Source: CAD feature listing. Evaluate the final solid. Frame: model axes, mm. Face numbers are marked on the shaded views. A direction names the side the tool comes from. Give positions to 0.01 mm unless a question says otherwise; leave off trailing zeros. Order: outer loops, then holes, each group sorted by start corner. A loop starts at its lowest first (then second) coordinate and runs counter-clockwise, first axis right, second up. Notation, with made-up numbers: M 78.5,-13.5 L 94.5,-13.5 A37 cw 94.5,24.5 Z; hole C 49,0 d8. An arc over 180 degrees is marked long. Answer as a JSON object with one key per item and string values. Group by question number.
1. Pin query (flat end, axial travel): P1, Ø2, axis at x = -6.5, y = 9.5, coming from the +Z side; P2, Ø4, axis at y = 6, z = 14, coming from the +X side; P3, Ø1, axis at x = -8, z = 10.5, coming from the +Y side. Return the tip coordinate at first contact, or that it passes through.
2. Set-up query: the marked faces 4 and 5. Return all of +Z, -Z, +X, -X, +Y, -Y with unobstructed straight access to the full face (end or side cutting, diameter ignored); none if empty.
3. Section query D-D (x = -18). Output: boundary loops of the cut face in (y, z).
4. Section query A-A (y = 0). Output: boundary loops of the cut face in (x, z), plus the area to 4 significant figures.
5. Material intervals for L1, parallel to Y at x = 0, z = 5.5; L2, parallel to Z at x = 0, y = -5; L3, parallel to Z at x = -7.5, y = -7, sorted ascending. Write a range as [from, to].
6. Section query C-C (z = 16.75). Output: boundary loops of the cut face in (x, y), plus the area to 3 significant figures.
7. Pull-direction query (X, two-part tool) for the marked faces 1, 2 and 3; classes: +X half, -X half, draft (parallel to the pull), parting line (faces both ways), or undercut.
from build123d import *

# Parameters (mm, degrees)
SKETCH_1_R          = 22.5
EXTRUDE_1_DEPTH     = 13.5
SKETCH_2_R          = 9
EXTRUDE_2_DEPTH     = 7
SKETCH_3_R          = 4
CUT_EXTRUDE_1_DEPTH = 38.851684243
SKETCH_4_R          = 1.5
CUT_EXTRUDE_2_DEPTH = 38.851684243
SKETCH_5_R          = 1.5
CUT_EXTRUDE_3_DEPTH = 38.851684297


with BuildPart() as part:
    # 스케치1 → 보스-돌출1 (new body)
    with BuildSketch(Plane.XY):
        Circle(SKETCH_1_R)
    extrude(amount=EXTRUDE_1_DEPTH)

    # 스케치2 → 보스-돌출2 (add)
    with BuildSketch(Plane.XY.offset(13.5)):
        Circle(SKETCH_2_R)
    extrude(amount=EXTRUDE_2_DEPTH)

    # 스케치3 → 컷-돌출1 (cut, through all)
    with BuildSketch(Plane.XY.offset(20.5)):
        Circle(SKETCH_3_R)
    extrude(amount=-CUT_EXTRUDE_1_DEPTH, mode=Mode.SUBTRACT)

    # 스케치4 → 컷-돌출2 (cut, through all)
    with BuildSketch(Plane(origin=(0, 0, 0), x_dir=(1, 0, 0), z_dir=(0, 1, 0))):
        with Locations(Location((0, -17.5, 0), (0, 0, 270))):
            Circle(SKETCH_4_R)
    extrude(amount=-CUT_EXTRUDE_2_DEPTH, mode=Mode.SUBTRACT)

    # 스케치5 → 컷-돌출3 (cut, through all)
    with BuildSketch(Plane(origin=(0, 0, 0), x_dir=(0, 0, -1), z_dir=(1, 0, 0))):
        with Locations((-17.5, 0)):
            Circle(SKETCH_5_R)
    extrude(amount=-CUT_EXTRUDE_3_DEPTH, mode=Mode.SUBTRACT)


solid = part.part
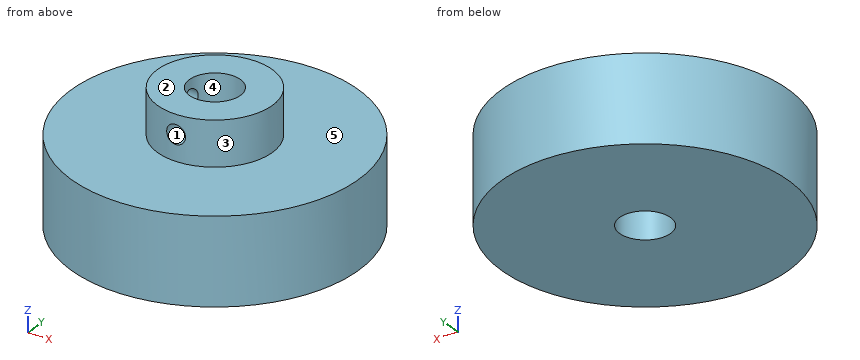
Answer sheet:
{
 "1": {"P1": "z = 13.5", "P2": "x = 22.13", "P3": "y = 21.21"},
 "2": {"face 4": "+Z, -Z", "face 5": "+Z"},
 "3": {"outline": "M -13.5,0 L 13.5,0 L 13.5,13.5 L -13.5,13.5 Z"},
 "4": {"outline": "M -22.5,0 L -4,0 L -4,16 L -9,16 L -9,13.5 L -22.5,13.5 Z; M -9,19 L -4,19 L -4,20.5 L -9,20.5 Z; M 4,0 L 22.5,0 L 22.5,13.5 L 9,13.5 L 9,20.5 L 4,20.5 Z", "area": "554.5 mm^2"},
 "5": {"L1": "[-22.5, -4], [4, 22.5]", "L2": "[0, 16], [19, 20.5]", "L3": "[0, 13.5]"},
 "6": {"outline": "M -8.91,-1.3 A9 ccw -1.3,-8.91 L -1.3,-3.78 A4 cw -3.78,-1.3 Z; M -8.91,1.3 L -3.78,1.3 A4 cw long 1.3,-3.78 L 1.3,-8.91 A9 ccw long Z", "area": "178 mm^2"},
 "7": {"face 1": "undercut", "face 2": "draft", "face 3": "parting line"}
}
